CAD build for the part. Positions are in the model's coordinates, mm. A direction names the side the tool comes from. Round coordinates to 2 decimals unless told otherwise and drop trailing zeros. Order: outer loops, then holes, each group sorted by start corner. A loop starts at its lowest first (then second) coordinate and runs counter-clockwise, first axis right, second up. Notation, with made-up numbers: M 21.25,55 L 53.25,55 A17 cw 53.25,80 Z; hole C 56.5,30.5 d5. An arc over 180 degrees is marked long. Put each result on its own line as item: value.
```python
from build123d import *

# Parameters (mm, degrees)
SKETCH1_R           = 45
BOSS_EXTRUDE1_DEPTH = 2
SKETCH3_R           = 1.75
CUT_EXTRUDE1_DEPTH  = 64.671029519
SKETCH4_W           = 21
SKETCH4_H           = 12
CUT_EXTRUDE2_DEPTH  = 64.671029519


with BuildPart() as part:
    # Sketch1 → Boss-Extrude1 (new body)
    with BuildSketch(Plane(origin=(0, 0, 0), x_dir=(1, 0, 0), z_dir=(0, 1, 0))):
        with Locations(Location((0, 0, 0), (0, 0, 270))):
            Circle(SKETCH1_R)
    extrude(amount=BOSS_EXTRUDE1_DEPTH)

    # Sketch3 → Cut-Extrude1 (cut, through all)
    with BuildSketch(Plane(origin=(0, 2, 0), x_dir=(1, 0, 0), z_dir=(0, 1, 0))):
        with Locations(Location((0, 40, 0), (0, 0, 270))):
            Circle(SKETCH3_R)
        with Locations(Location((40, 0, 0), (0, 0, 270))):
            Circle(SKETCH3_R)
        with Locations(Location((0, -40, 0), (0, 0, 270))):
            Circle(SKETCH3_R)
        with Locations(Location((-40, 0, 0), (0, 0, 270))):
            Circle(SKETCH3_R)
    extrude(amount=-CUT_EXTRUDE1_DEPTH, mode=Mode.SUBTRACT)

    # Sketch4 → Cut-Extrude2 (cut, through all)
    with BuildSketch(Plane(origin=(0, 2, 0), x_dir=(1, 0, 0), z_dir=(0, 1, 0))):
        Rectangle(SKETCH4_W, SKETCH4_H)
    extrude(amount=-CUT_EXTRUDE2_DEPTH, mode=Mode.SUBTRACT)


solid = part.part
```
Item 1: Band-saw the part on B-B on x = 0. Give the cut face in (y, z).
Answers below:
outline: M 0,-45 L 2,-45 L 2,-41.75 L 0,-41.75 Z; M 0,-38.25 L 2,-38.25 L 2,-6 L 0,-6 Z; M 0,6 L 2,6 L 2,38.25 L 0,38.25 Z; M 0,41.75 L 2,41.75 L 2,45 L 0,45 Z
Item 2: Probe line 1 along X through (y, z) = (1.25, 0); line 2 along X through (y, z) = (0.7, 1.5) (3 decimals); line 3 along Z through (x, y) = (4.5, 1.45). List the from-to ranges inside material, lowest first. Write a range as [from, to].
Answers below:
line 1: [-45, -41.75], [-38.25, -10.5], [10.5, 38.25], [41.75, 45]
line 2: [-44.975, -40.901], [-39.099, -10.5], [10.5, 39.099], [40.901, 44.975]
line 3: [-44.77, -6], [6, 44.77]
Item 3: Pin check, flat tips, straight feed: P1, Ø3, axis at x = 40, z = 0, coming from the -Y side; P2, Ø1, axis at y = 1, z = 1, coming from the +X side; P3, Ø0.6, axis at x = -3.5, y = 1, coming from the -Z side. Stop position of each tip, or through.
Answers below:
P1: through
P2: x = 45
P3: z = -44.89
Item 4: Mould opens along X. For faces 3 (the cylindrical face through (-0.67, 1.014, 41.617)), 4 (the cylindrical face through (-17.235, 0.986, 41.569)), 5 (the flat face through (1, 2, 9)) say: pulls with the +X half, pulls with the -X half, needs draft (parallel to the pull), parting line crosses it, or undercut.
Answers below:
face 3: undercut
face 4: parting line crosses it
face 5: needs draft
Item 5: Tool access for faces 1 (the flat face through (0, 1, -6)), 2 (the flat face through (1, 0, 9)): list every direction of +Z, -Z, +X, -X, +Y, -Y with a clear straight run to the whole face (end or side of a thin tool).
Answers below:
face 1: +Y, -Y
face 2: +Z, -Z, +X, -X, -Y
Item 6: Band-saw the part on C-C on z = 40. Give the cut face in (x, y), and give its area (3 significant figures).
Answers below:
outline: M -20.62,0 L -1.75,0 L -1.75,2 L -20.62,2 Z; M 1.75,0 L 20.62,0 L 20.62,2 L 1.75,2 Z
area: 75.5 mm²
Item 7: Band-saw the part on D-D on z = 0. Give the cut face in (x, y), and give its area (3 significant figures).
Answers below:
outline: M -45,0 L -41.75,0 L -41.75,2 L -45,2 Z; M -38.25,0 L -10.5,0 L -10.5,2 L -38.25,2 Z; M 10.5,0 L 38.25,0 L 38.25,2 L 10.5,2 Z; M 41.75,0 L 45,0 L 45,2 L 41.75,2 Z
area: 124 mm²
Item 8: Band-saw the part on A-A on y = 1.6. Give the cut face in (x, z), and give its area (3 significant figures).
Answers below:
outline: C 0,0 d90; hole C -40,0 d3.5; hole M -10.5,-6 L 10.5,-6 L 10.5,6 L -10.5,6 Z; hole C 0,-40 d3.5; hole C 0,40 d3.5; hole C 40,0 d3.5
area: 6,070 mm²
